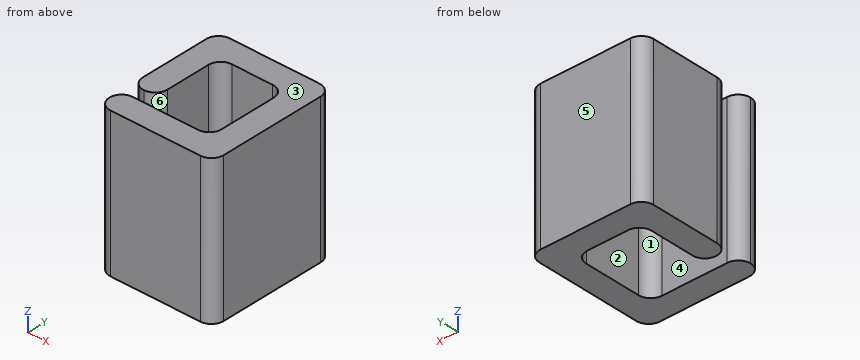
```python
from build123d import *

# Parameters (mm, degrees)
F0_W     = 14
F0_H     = 18
F1_DEPTH = 3
F2_W     = 3
F2_H     = 8.5
F2_H_2   = 10
F3_DEPTH = 18
F4_R     = 1.49999


# Not quite as in the source:
# - a fillet or chamfer is up to 0.001 mm smaller than in the source, because OpenCascade refuses the exact size


with BuildPart() as f1:
    # F0 (on Front) → F1 (new body)
    with BuildSketch(Plane.XZ):
        with Locations((7, 9)):
            Rectangle(F0_W, F0_H)
    extrude(amount=F1_DEPTH)

    # F2 (on face) → F3 (join, through all)
    with BuildSketch(Plane.XY.offset(18)):
        with Locations((1.5, -7.25)):
            Rectangle(F2_W, F2_H)
        Polygon((3, -13), (0, -13), (0, -16), (14, -16), (14, -13), (11, -13), align=None)
        with Locations((12.5, -8)):
            Rectangle(F2_W, F2_H_2)
    extrude(amount=-F3_DEPTH)

    # F4 (radius 1.5 in the source; OpenCascade refuses exactly that, so slightly less here)
    f4_edges = [f1.edges().sort_by_distance(p)[0] for p in [
        (0, -11.5, 9),
        (0, -13, 9),
        (0, -16, 9),
        (3, -11.5, 9),
        (14, -16, 9),
        (14, 0, 9),
        (0, 0, 9),
        (3, -3, 9),
        (11, -3, 9),
        (11, -13, 9),
    ]]
    fillet(f4_edges, radius=F4_R)


solid = f1.part
```
CAD build for the part. Positions are in the model's coordinates, mm. Face numbers are marked on the shaded views. A direction names the side the tool comes from. Give positions to 0.01 mm unless a question says otherwise; leave off trailing zeros. Loops run counter-clockwise (first coordinate to the right, second up) from the corner with the lowest first, then second, coordinate; pieces in that order, holes last. Notation, with made-up numbers: M 76.5,71.5 L 104.5,71.5 A25 cw 104.5,87.5 Z; hole C -31.5,72 d10. An arc over 180 degrees is marked long. Use one line per item in the form item = value.
Item 1: Slice it at D-D (y = -12). List the corners of the cut face in (x, z), plus the area to 3 significant figures.
Determined:
outline = M 10.91,0 L 14,0 L 14,18 L 10.91,18 Z
area = 55.5 mm2
Item 2: Drill centre lines: probe 1 along X at (y, z) = (-9.5, 11.75); probe 2 along Y at (x, z) = (9.5, 8.5); probe 3 along Y at (x, z) = (3.5, 8.25). Where is each one in solid material? Low to high. Write a range as from..to.
Determined:
probe_1 = 0..3, 11..14
probe_2 = -16..-13, -3..0
probe_3 = -16..-13, -3.38..0
Item 3: Slice it at A-A (y = -9.25). List the corners of the cut face in (x, z).
Determined:
outline = M 0,0 L 3,0 L 3,18 L 0,18 Z; M 11,0 L 14,0 L 14,18 L 11,18 Z
Item 4: Slice it at B-B (x = 7). List the corners of the cut face in (y, z).
Determined:
outline = M -16,0 L -13,0 L -13,18 L -16,18 Z; M -3,0 L 0,0 L 0,18 L -3,18 Z
Item 5: Which spindle directions (+Z, -Z, +X, -X, +Y, -Y) get a long thin tool onto all of the face, cutting with end or side? Do the marked faces 4, 5 and 6. Say none if no direction does.
Determined:
face_4 = +Z, -Z, -X
face_5 = +Z, -Z, +X, -X, +Y
face_6 = +Z, -Z
Item 6: Flat gauge pin, fed straight in: pin 1 (1 mm diameter, centred on x = 12.5, y = -9, fed in from -Z). Where does the tip first touch, or does it go through?
Determined:
pin_1 = 0
Item 7: Two-plate mould, pull along X, no slides. Class the marked faces 1, 2 and 3: pulls with the +X half, pulls with the -X half, needs draft (parallel to the pull), parting line crosses it, or undercut.
Determined:
face_1 = pulls with the -X half
face_2 = undercut
face_3 = needs draft
